Geometry: final body of the model. Coordinates: model frame, mm. A direction names the side the tool comes from. Give positions to 0.01 mm unless a question says otherwise; leave off trailing zeros. Loops run counter-clockwise (first coordinate to the right, second up) from the corner with the lowest first, then second, coordinate; pieces in that order, holes last.
from build123d import *

# Parameters (mm, degrees)
ESBO_O1_W                = 112
ESBO_O1_H                = 96
RESSALTO_EXTRUS_O1_DEPTH = 2
ESBO_O2_W                = 108
ESBO_O2_H                = 3
ESBO_O2_H_2              = 82
RESSALTO_EXTRUS_O2_DEPTH = 40
ESBO_O3_W                = 104
ESBO_O3_H                = 38
CORTE_EXTRUS_O1_DEPTH    = 154.37535656
ESBO_O4_W                = 52
ESBO_O4_H                = 30
RESSALTO_EXTRUS_O3_DEPTH = 11.5
ESBO_O5_W                = 46
ESBO_O5_H                = 26
CORTE_EXTRUS_O2_DEPTH    = 12
ESBO_O6_W                = 43.2
ESBO_O6_H                = 26
CORTE_EXTRUS_O3_DEPTH    = 1.5
RESSALTO_EXTRUS_O4_DEPTH = 26
ESBO_O8_W                = 5.4
ESBO_O8_H                = 8.6
RESSALTO_EXTRUS_O5_DEPTH = 5.6
CORTE_EXTRUS_O4_DEPTH    = 8.6
CORTE_EXTRUS_O5_DEPTH    = 8.6
CORTE_EXTRUS_O6_DEPTH    = 8.6
CORTE_EXTRUS_O7_DEPTH    = 6.6
FILETE1_R                = 0.5
FILETE2_R                = 0.5
CORTE_EXTRUS_O8_DEPTH    = 2
ESBO_O16_R               = 1.5
CORTE_EXTRUS_O9_DEPTH    = 2
ESBO_O17_R               = 1.5
CORTE_EXTRUS_O10_DEPTH   = 154.37535656


with BuildPart() as part:
    # Esboço1 → Ressalto-extrusão1 (new body)
    with BuildSketch(Plane(origin=(0, 0, 0), x_dir=(1, 0, 0), z_dir=(0, 1, 0))):
        with Locations((56, 48)):
            Rectangle(ESBO_O1_W, ESBO_O1_H)
    extrude(amount=RESSALTO_EXTRUS_O1_DEPTH)

    # Esboço2 → Ressalto-extrusão2 (add)
    with BuildSketch(Plane(origin=(0, 2, 0), x_dir=(1, 0, 0), z_dir=(0, 1, 0))):
        Polygon((0, 96), (2, 96), (110, 96), (112, 96), (112, 0), (110, 0), (2, 0), (0, 0), align=None)
        with Locations((56, 92.5)):
            Rectangle(ESBO_O2_W, ESBO_O2_H, mode=Mode.SUBTRACT)
        with Locations((56, 3.5)):
            Rectangle(ESBO_O2_W, ESBO_O2_H, mode=Mode.SUBTRACT)
        with Locations((56, 48)):
            Rectangle(ESBO_O2_W, ESBO_O2_H_2, mode=Mode.SUBTRACT)
    extrude(amount=RESSALTO_EXTRUS_O2_DEPTH)

    # Esboço3 → Corte-extrusão1 (cut, through all)
    with BuildSketch(Plane.XY):
        with Locations((56, 23)):
            Rectangle(ESBO_O3_W, ESBO_O3_H)
    extrude(amount=-CORTE_EXTRUS_O1_DEPTH, mode=Mode.SUBTRACT)

    # Esboço4 → Ressalto-extrusão3 (add)
    with BuildSketch(Plane(origin=(2, 0, 0), x_dir=(0, 0, -1), z_dir=(1, 0, 0))):
        with Locations((31, 17)):
            Rectangle(ESBO_O4_W, ESBO_O4_H)
    extrude(amount=RESSALTO_EXTRUS_O3_DEPTH)

    # Esboço5 → Corte-extrusão2 (cut)
    with BuildSketch(Plane.ZY):
        with Locations((-31, 16)):
            Rectangle(ESBO_O5_W, ESBO_O5_H)
    extrude(amount=-CORTE_EXTRUS_O2_DEPTH, mode=Mode.SUBTRACT)

    # Esboço6 → Corte-extrusão3 (cut)
    with BuildSketch(Plane.ZY.offset(-12)):
        with Locations((-31, 16)):
            Rectangle(ESBO_O6_W, ESBO_O6_H)
    extrude(amount=-CORTE_EXTRUS_O3_DEPTH, mode=Mode.SUBTRACT)

    # Esboço7 → Ressalto-extrusão4 (add)
    with BuildSketch(Plane(origin=(0, 3, 0), x_dir=(1, 0, 0), z_dir=(0, 1, 0))):
        Polygon((12, 52.6), (12, 53.6), (11, 52.6), align=None)
        Polygon((12, 9.4), (12, 8.4), (11, 9.4), align=None)
    extrude(amount=RESSALTO_EXTRUS_O4_DEPTH)

    # Esboço8 → Ressalto-extrusão5 (add)
    with BuildSketch(Plane(origin=(13.5, 0, 0), x_dir=(0, 0, -1), z_dir=(1, 0, 0))):
        with Locations((10.1, 16)):
            Rectangle(ESBO_O8_W, ESBO_O8_H)
        with Locations((51.9, 16)):
            Rectangle(ESBO_O8_W, ESBO_O8_H)
    extrude(amount=RESSALTO_EXTRUS_O5_DEPTH)

    # Esboço9 → Corte-extrusão4 (cut)
    with BuildSketch(Plane(origin=(0, 20.3, 0), x_dir=(1, 0, 0), z_dir=(0, 1, 0))):
        Polygon((13.5, 54.6), (19.1, 52.8), (19.1, 54.6), align=None)
        Polygon((13.5, 7.4), (19.1, 7.4), (19.1, 9.2), align=None)
    extrude(amount=-CORTE_EXTRUS_O4_DEPTH, mode=Mode.SUBTRACT)

    # Esboço10 → Corte-extrusão5 (cut)
    with BuildSketch(Plane(origin=(0, 20.3, 0), x_dir=(1, 0, 0), z_dir=(0, 1, 0))):
        Polygon((13.5, 12.8), (16, 12.8), (13.5, 9.8), align=None)
        Polygon((13.5, 49.2), (16, 49.2), (13.5, 52.2), align=None)
    extrude(amount=-CORTE_EXTRUS_O5_DEPTH, mode=Mode.SUBTRACT)

    # Esboço11 → Corte-extrusão6 (cut)
    with BuildSketch(Plane(origin=(0, 20.3, 0), x_dir=(1, 0, 0), z_dir=(0, 1, 0))):
        Polygon((19.1, 49.2), (18, 49.2), (18, 49.7), (19.1, 51.2), align=None)
        Polygon((19.1, 12.8), (18, 12.8), (18, 12.3), (19.1, 10.8), align=None)
    extrude(amount=-CORTE_EXTRUS_O6_DEPTH, mode=Mode.SUBTRACT)

    # Esboço14 → Corte-extrusão7 (cut)
    with BuildSketch(Plane(origin=(0, 19.3, 0), x_dir=(1, 0, 0), z_dir=(0, 1, 0))):
        Polygon((18, 12.3), (18, 10.5), (18.5, 10.5), (19.033236994, 10.891040462), align=None)
        Polygon((18, 49.7), (18, 51.5), (18.5, 51.5), (19.033236994, 51.108959538), align=None)
    extrude(amount=-CORTE_EXTRUS_O7_DEPTH, mode=Mode.SUBTRACT)

    # Filete1
    filete1_edges = [part.edges().sort_by_distance(p)[0] for p in [
        (16.3, 11.7, -53.7),
        (19.1, 16, -52.8),
        (16.3, 20.3, -53.7),
    ]]
    fillet(filete1_edges, radius=FILETE1_R)

    # Filete2
    filete2_edges = [part.edges().sort_by_distance(p)[0] for p in [
        (16.3, 11.7, -8.3),
        (19.1, 16, -9.2),
        (16.3, 20.3, -8.3),
    ]]
    fillet(filete2_edges, radius=FILETE2_R)

    # Esboço15 → Corte-extrusão8 (cut)
    with BuildSketch(Plane(origin=(112, 0, 0), x_dir=(0, 0, -1), z_dir=(1, 0, 0))):
        with BuildLine():
            Line((21.4, 5), (42.6, 5))
            ThreePointArc((42.6, 5), (44.721320344, 5.878679656), (45.6, 8))
            Line((45.6, 8), (45.6, 21.2))
            ThreePointArc((45.6, 21.2), (44.721320344, 23.321320344), (42.6, 24.2))
            Line((42.6, 24.2), (21.4, 24.2))
            ThreePointArc((21.4, 24.2), (19.278679656, 23.321320344), (18.4, 21.2))
            Line((18.4, 21.2), (18.4, 8))
            ThreePointArc((18.4, 8), (19.278679656, 5.878679656), (21.4, 5))
        make_face()
    extrude(amount=-CORTE_EXTRUS_O8_DEPTH, mode=Mode.SUBTRACT)

    # Esboço16 → Corte-extrusão9 (cut)
    with BuildSketch(Plane(origin=(112, 0, 0), x_dir=(0, 0, -1), z_dir=(1, 0, 0))):
        with Locations((52, 14.6)):
            Circle(ESBO_O16_R)
        with Locations((12, 14.6)):
            Circle(ESBO_O16_R)
    extrude(amount=-CORTE_EXTRUS_O9_DEPTH, mode=Mode.SUBTRACT)

    # Esboço17 → Corte-extrusão10 (cut, through all)
    with BuildSketch(Plane.ZY):
        with Locations((-78, 37)):
            Circle(ESBO_O17_R)
        with Locations((-18, 37)):
            Circle(ESBO_O17_R)
    extrude(amount=-CORTE_EXTRUS_O10_DEPTH, mode=Mode.SUBTRACT)


solid = part.part
Item 1: Ray query, probe 1 along Y at (x, z) = (1.2, -18); probe 2 along X at (y, z) = (37.5, -66); probe 3 along X at (y, z) = (30.5, -35.5). Return the intervals inside material, ascending.
Values follow:
probe 1: y = 0 to 3, 29 to 35.5, 38.5 to 42
probe 2: x = 0 to 2, 110 to 112
probe 3: x = 0 to 13.5, 110 to 112
Item 2: Set-up query: faces 1 (the face through (2, 22, -92)), 2 (the face through (16, 20.3, -10)), 3 (the face through (7, 3, -31)), 4 (the face through (16, 11.7, -52)). Return all of +Z, -Z, +X, -X, +Y, -Y with unobstructed straight access to the full face (end or side cutting, diameter ignored); none if empty.
Values follow:
face 1: +Y
face 2: +Z, -Z, +Y
face 3: -X
face 4: +Z, -Z
Item 3: Section query C-C on x = 89.5. Return loops of the section in (y, z), plus the area to 3 significant figures.
Values follow:
outline: (0, -96) - (4, -96) - (4, -94) - (2, -94) - (2, -91) - (4, -91) - (4, -89) - (2, -89) - (2, -7) - (4, -7) - (4, -5) - (2, -5) - (2, -2) - (4, -2) - (4, 0) - (0, 0) - close
area: 208 mm2
Item 4: Pin query (flat end, axial travel): pin 1 (1 mm diameter, centred on x = 41.5, z = -6.5, fed in from +Y); pin 2 (1.5 mm diameter, centred on y = 15.5, z = -93, fed in from -X); pin 3 (6 mm diameter, centred on x = 8, y = 18.5, fed in from -Z); pin 4 (6 mm diameter, centred on x = 14, z = -47, fed in from +Y). Return the tip coordinate at first contact, or that it passes through.
Values follow:
pin 1: stops at y = 4
pin 2: stops at x = 0
pin 3: stops at z = -57
pin 4: stops at y = 32
Item 5: Section query A-A on z = -78. Return loops of the section in (x, y), plus the area to 3 significant figures.
Values follow:
outline: (0, 0) - (112, 0) - (112, 35.5) - (110, 35.5) - (110, 2) - (2, 2) - (2, 35.5) - (0, 35.5) - close; (0, 38.5) - (2, 38.5) - (2, 42) - (0, 42) - close; (110, 38.5) - (112, 38.5) - (112, 42) - (110, 42) - close
area: 372 mm2
Item 6: Section query B-B on y = 37. Give the number of separate pieces and of enclosed holes in the cut face, plus the area to 3 significant figures.
Values follow:
separate pieces: 6
enclosed holes: 0
area: 392 mm2
Item 7: Draft query along Z for faces 5 (the face through (16.163, 16.053, -8.256)), 6 (the face through (16, 11.7, -10)), 7 (the face through (12, 16, -52.6)). Return one class per face: +Z half, -Z half, draft (parallel to the pull), parting line (faces both ways), or undercut.
Values follow:
face 5: +Z half
face 6: draft
face 7: undercut
